Part model, mm, in its own coordinate system. A direction names the side the tool comes from. Coordinates: 2 decimals unless noted, no trailing zeros. Loops run counter-clockwise (first coordinate to the right, second up) from the corner with the lowest first, then second, coordinate; pieces in that order, holes last.
```python
from build123d import *

# Parameters (mm, degrees)
EXTRUDE_1_DEPTH       = 200
SKETCH_3_W            = 148
SKETCH_3_H            = 194
CUT_EXTRUDE_1_DEPTH   = 44
SKETCH_4_W            = 8
SKETCH_4_H            = 194
EXTRUDE_1_2_DEPTH     = 44
CUT_EXTRUDE_2_DEPTH   = 222.580685079
CUT_EXTRUDE_5_DEPTH   = 219.876677606
MOVE_FACE_1_BY        = 2
MOVE_FACE_1_2_BY      = 2
CUT_EXTRUDE_6_DEPTH   = 222.580685079
CUT_EXTRUDE_7_DEPTH   = 16.595837
MOVE_FACE_2_BY        = 45
MOVE_FACE_3_BY        = 20
SKETCH_13_W           = 71
SKETCH_13_H           = 47
CUT_EXTRUDE_8_DEPTH   = 25
SKETCH_14_W           = 69
SKETCH_14_H           = 26
CUT_EXTRUDE_9_DEPTH   = 45
CUT_EXTRUDE_10_DEPTH  = 45
CHAMFER_1_SIZE        = 25
CUT_EXTRUDE_11_REACH  = 222.964
SKETCH_16_W           = 71
SKETCH_16_H           = 85
SKETCH_17_W           = 71
SKETCH_17_H           = 3
EXTRUDE_2_DEPTH       = 10
SKETCH_18_W           = 18.7
SKETCH_18_H           = 5
CUT_EXTRUDE_12_DEPTH  = 2.2
SKETCH_19_W           = 69
SKETCH_19_H           = 90
EXTRUDE_3_DEPTH       = 15
SKETCH_20_W           = 56
SKETCH_20_H           = 87
CUT_EXTRUDE_13_DEPTH  = 10
CUT_EXTRUDE_14_REACH  = 220.472
SKETCH_21_W           = 36
SKETCH_21_H           = 34
SKETCH_22_W           = 2
SKETCH_22_H           = 17
SKETCH_22_H_2         = 35
CUT_EXTRUDE_1_2_DEPTH = 7
MOVE_FACE_4_BY        = 3
CHAMFER_2_SIZE        = 1


with BuildPart() as part:
    # 草图1 → Extrude 1 (new body)
    with BuildSketch(Plane.XY):
        Polygon((77, 0), (-77, 0), (-77, 31), (-83, 37), (-83, 41), (-77, 47), (77, 47), (83, 41), (83, 37), (77, 31), align=None)
    extrude(amount=-EXTRUDE_1_DEPTH)

    # 草图3 → Cut-Extrude 1 (cut)
    with BuildSketch(Plane(origin=(0, 47, 0), x_dir=(1, 0, 0), z_dir=(0, 1, 0))):
        with Locations((0, 100)):
            Rectangle(SKETCH_3_W, SKETCH_3_H)
    extrude(amount=-CUT_EXTRUDE_1_DEPTH, mode=Mode.SUBTRACT)

    # 草图4 → Extrude 1 2 (add)
    with BuildSketch(Plane(origin=(0, 3, 0), x_dir=(1, 0, 0), z_dir=(0, 1, 0))):
        with Locations((1, 100)):
            Rectangle(SKETCH_4_W, SKETCH_4_H)
    extrude(amount=EXTRUDE_1_2_DEPTH)

    # 草图5 → 切除-拉伸2 (cut, through all)
    with BuildSketch(Plane(origin=(0, 0, -200), x_dir=(-1, 0, 0), z_dir=(0, 0, -1))):
        Polygon((-74, 47), (-74, 44.767409819), (-79, 39.767409819), (-79, 38.656854249), (-74, 33.656854249), (-74, 26), (-5, 26), (-5, 33.656854249), (0, 38.656854249), (0, 39.767409819), (-5, 44.767409819), (-5, 47), align=None)
    extrude(amount=-CUT_EXTRUDE_2_DEPTH, mode=Mode.SUBTRACT)

    # 草图9 → 切除-拉伸5 (cut, through all)
    with BuildSketch(Plane(origin=(0, 0, -3), x_dir=(-1, 0, 0), z_dir=(0, 0, -1))):
        Polygon((-4.404163056, 47), (3, 39.595836944), (74, 39.595836944), (74, 47), (3, 47), align=None)
    extrude(amount=CUT_EXTRUDE_5_DEPTH, mode=Mode.SUBTRACT)

    # Move Face 1: a face moved outward by 2.0
    extrude(part.faces().sort_by_distance((39.5, 14.5, -197))[0], amount=MOVE_FACE_1_BY, dir=(0, 0, 1))

    # Move Face 1 2: a face moved outward by 2.0
    extrude(part.faces().sort_by_distance((-38.5, 21.297918472, -197))[0], amount=MOVE_FACE_1_2_BY, dir=(0, 0, 1))

    # 草图11 → 切除-拉伸6 (cut, through all)
    with BuildSketch(Plane.XZ):
        Polygon((51.883419246, -200), (53.904145188, -196.5), (23.095854812, -196.5), (25.116580754, -200), align=None)
        Polygon((-53.904145188, -196.5), (-23.095854812, -196.5), (-25.116580754, -200), (-51.883419246, -200), align=None)
    extrude(amount=-CUT_EXTRUDE_6_DEPTH, mode=Mode.SUBTRACT)

    # 草图12 → 切除-拉伸7 (cut)
    with BuildSketch(Plane(origin=(0, 39.595836944, 0), x_dir=(1, 0, 0), z_dir=(0, 1, 0))):
        Polygon((-53.904145188, 196.5), (-51.883419246, 200), (-74, 200), (-74, 195), (-3, 195), (-3, 200), (-25.116580754, 200), (-23.095854812, 196.5), align=None)
        Polygon((53.904145188, 196.5), (23.095854812, 196.5), (25.116580754, 200), (5, 200), (5, 195), (74, 195), (74, 200), (51.883419246, 200), align=None)
    extrude(amount=-CUT_EXTRUDE_7_DEPTH, mode=Mode.SUBTRACT)

    # Move Face 2: a face moved outward by 45.0
    extrude(part.faces().sort_by_distance((-10.200110487, 20.43272532, 0))[0], amount=MOVE_FACE_2_BY, dir=(0, 0, 1))

    # Move Face 3: a face moved inward by 20.0
    extrude(part.faces().sort_by_distance((-38.169755743, 25.169887896, -3))[0], amount=MOVE_FACE_3_BY, dir=(0, 0, 1), mode=Mode.SUBTRACT)

    # 草图13 → 切除-拉伸8 (cut)
    with BuildSketch(Plane.XY.offset(45)):
        with Locations((-38.5, 23.5)):
            Rectangle(SKETCH_13_W, SKETCH_13_H)
    extrude(amount=-CUT_EXTRUDE_8_DEPTH, mode=Mode.SUBTRACT)

    # 草图14 → 切除-拉伸9 (cut)
    with BuildSketch(Plane.XY.offset(45)):
        with Locations((39.5, 13)):
            Rectangle(SKETCH_14_W, SKETCH_14_H)
    extrude(amount=-CUT_EXTRUDE_9_DEPTH, mode=Mode.SUBTRACT)

    # 草图15 → 切除-拉伸10 (cut)
    with BuildSketch(Plane.XY.offset(45)):
        Polygon((5, 0), (0, 0), (0, 25.656854249), (5, 30.656854249), align=None)
    extrude(amount=-CUT_EXTRUDE_10_DEPTH, mode=Mode.SUBTRACT)

    # 倒角1
    chamfer_1_edges = [part.edges().sort_by_distance(p)[0] for p in [
        (75.5, 0, 45),
        (-1.5, 0, 45),
        (-75.5, 0, 45),
    ]]
    chamfer(chamfer_1_edges, length=CHAMFER_1_SIZE)

    # 草图16 → 切除-拉伸11 (cut, up to next)
    with BuildSketch(Plane(origin=(0, 3, 0), x_dir=(1, 0, 0), z_dir=(0, 1, 0)), mode=Mode.PRIVATE) as cut_extrude_11_sk1:
        with Locations((-38.5, 152.5)):
            Rectangle(SKETCH_16_W, SKETCH_16_H)
    cut_extrude_11_tool1 = extrude(cut_extrude_11_sk1.sketch, amount=-CUT_EXTRUDE_11_REACH, mode=Mode.PRIVATE) & part.part
    add(cut_extrude_11_tool1.solids().sort_by_distance((-38.5, 3, -152.5))[0], mode=Mode.SUBTRACT)

    # 草图17 → 凸台-拉伸2 (add)
    with BuildSketch(Plane(origin=(0, 3, 0), x_dir=(1, 0, 0), z_dir=(0, 1, 0))):
        with Locations((-38.5, 108.5)):
            Rectangle(SKETCH_17_W, SKETCH_17_H)
    extrude(amount=EXTRUDE_2_DEPTH)

    # 草图18 → 切除-拉伸12 (cut)
    with BuildSketch(Plane(origin=(0, 23, 0), x_dir=(1, 0, 0), z_dir=(0, 1, 0))):
        with Locations((-12.35, 197.5)):
            Rectangle(SKETCH_18_W, SKETCH_18_H)
        with Locations((-64.65, 197.5)):
            Rectangle(SKETCH_18_W, SKETCH_18_H)
    extrude(amount=-CUT_EXTRUDE_12_DEPTH, mode=Mode.SUBTRACT)

    # 草图19 → 凸台-拉伸3 (add)
    with BuildSketch(Plane(origin=(0, 3, 0), x_dir=(1, 0, 0), z_dir=(0, 1, 0))):
        with Locations((39.5, 150)):
            Rectangle(SKETCH_19_W, SKETCH_19_H)
    extrude(amount=EXTRUDE_3_DEPTH)

    # 草图20 → 切除-拉伸13 (cut)
    with BuildSketch(Plane(origin=(0, 18, 0), x_dir=(1, 0, 0), z_dir=(0, 1, 0))):
        with Locations((33, 151.5)):
            Rectangle(SKETCH_20_W, SKETCH_20_H)
    extrude(amount=-CUT_EXTRUDE_13_DEPTH, mode=Mode.SUBTRACT)

    # 切除-拉伸14: up to this face of the body (flat: up to its plane)
    cut_extrude_14_end = Plane(part.part.faces().sort_by_distance((39.5, 3, -54))[0])
    # 草图21 → 切除-拉伸14 (cut, up to the picked face)
    with BuildSketch(Plane(origin=(0, 18, 0), x_dir=(1, 0, 0), z_dir=(0, 1, 0)), mode=Mode.PRIVATE) as cut_extrude_14_sk1:
        with Locations((33, 108)):
            Rectangle(SKETCH_21_W, SKETCH_21_H)
    cut_extrude_14_tool1 = split(extrude(cut_extrude_14_sk1.sketch, amount=-CUT_EXTRUDE_14_REACH, mode=Mode.PRIVATE), bisect_by=cut_extrude_14_end, keep=Keep.BOTH, mode=Mode.PRIVATE)
    add(cut_extrude_14_tool1.solids().sort_by(Axis((33, 18, -108), (0, -1, 0)))[0], mode=Mode.SUBTRACT)

    # 草图22 → Cut-Extrude 1 2 (cut)
    with BuildSketch(Plane(origin=(0, 18, 0), x_dir=(1, 0, 0), z_dir=(0, 1, 0))):
        with Locations((66, 181.5)):
            Rectangle(SKETCH_22_W, SKETCH_22_H)
        with Locations((66, 158.5)):
            Rectangle(SKETCH_22_W, SKETCH_22_H)
        with Locations((66, 126.5)):
            Rectangle(SKETCH_22_W, SKETCH_22_H_2)
    extrude(amount=-CUT_EXTRUDE_1_2_DEPTH, mode=Mode.SUBTRACT)

    # Move Face 4: a face moved outward by 3.0
    extrude(part.faces().sort_by_distance((66, 11, -126.5))[0], amount=MOVE_FACE_4_BY, dir=(0, 1, 0))

    # 倒角2
    chamfer_2_edges = [part.edges().sort_by_distance(p)[0] for p in [
        (-80, 34, 45),
        (-83, 39, 45),
        (-80, 44, 45),
        (80, 44, 45),
        (83, 39, 45),
        (80, 34, 45),
        (80, 34, -200),
        (83, 39, -200),
        (80, 44, -200),
        (-80, 44, -200),
        (-83, 39, -200),
        (-80, 34, -200),
        (2.5, 42.267409819, 45),
        (0, 39.212132034, 45),
        (2.5, 36.156854249, 45),
        (76.5, 36.156854249, 45),
        (79, 39.212132034, 45),
        (76.5, 42.267409819, 45),
        (76.5, 42.267409819, -200),
        (76.5, 36.156854249, -200),
        (2.5, 36.156854249, -200),
        (0, 39.212132034, -200),
        (2.5, 42.267409819, -200),
    ]]
    chamfer(chamfer_2_edges, length=CHAMFER_2_SIZE)


solid = part.part
```
Q1. Tool access for faces 5 (the flat face through (77, 16, -79)), 6 (the flat face through (76.545, 35.485, -199.507)), 7 (the flat face through (-65, 20.8, -198)), 8 (the flat face through (2.4, 35.56, 44.49)), 9 (the flat face through (31, 16, -195)): list every direction of +Z, -Z, +X, -X, +Y, -Y with a clear straight run to the whole face (end or side of a thin tool).
Q2. Saw through at D-D (x = -33). List the corners of the cut face in (y, z), plus the area to 4 significant figures.
Q3. Probe line 1 (X direction, y = 25.5, z = -134); line 2 (X direction, y = 10, z = -187); line 3 (Z direction, x = 33.5, y = 13.5). List the from-to ranges inside material, lowest first.
Q4. Saw through at C-C (z = -87). List the corners of the cut face in (x, y), plus the area to 3 significant figures.
Q5. Saw through at B-B (x = 9). List the corners of the cut face in (y, z).
Q6. Saw through at A-A (x = -11.5). List the corners of the cut face in (y, z), plus the area to 3 significant figures.
Q7. Drop flat-ended pins along their axis: P1, Ø0.6, axis at x = 66, z = -162, coming from the +Y side; P2, Ø1.1, axis at y = 46, z = -17.5, coming from the +X side; P3, Ø7, axis at x = 34.5, y = 13, coming from the -Z side; P4, Ø12, axis at x = -9.5, z = -123, coming from the -Y side. Give the stop position or say it passes through.
Q8. Mould opens along Z. For faces 1 (the flat face through (0, 13, -200)), 2 (the flat face through (-79.345, 43.958, 44.493)), 3 (the flat face through (0.754, 43.35, -93.019)), 4 (the flat face through (-39, 7, -110)) say: released by +Z, released by -Z, zero draft, split by the parting line, or undercut.
Checked values:
1. face 5: +Z, -Z, +X, -Y
1. face 6: -Z
1. face 7: -Z, +Y
1. face 8: +Z
1. face 9: +Y
2. outline: (0, -196.5) - (23, -196.5) - (23, -195) - (0, -195) - close; (0, -110) - (13, -110) - (13, -107) - (3, -107) - (3, 17) - (47, 17) - (47, 20) - (0, 20) - close
2. area: 586.5 mm2
3. line 1: x = -77 to -74, -3 to 5, 74 to 77
3. line 2: x = -77 to -74, -3 to 5, 61 to 77
3. line 3: z = -196.5 to -195, -3 to 0
4. outline: (-83, 37) - (-77, 31) - (-77, 0) - (77, 0) - (77, 31) - (83, 37) - (83, 41) - (77, 47) - (74, 47) - (74, 44.77) - (79, 39.77) - (79, 38.66) - (74, 33.66) - (74, 3) - (5, 3) - (5, 33.66) - (0, 38.66) - (0, 39.77) - (5, 44.77) - (5, 47) - (4.4, 47) - (-3, 39.6) - (-3, 3) - (-74, 3) - (-74, 47) - (-77, 47) - (-83, 41) - close
4. area: 1,110 mm2
5. outline: (0, -200) - (23, -200) - (23, -195) - (8, -195) - (8, -108) - (18, -108) - (18, -105) - (3, -105) - (3, -3) - (26, -3) - (26, 0) - (0, 0) - close
6. outline: (0, -200) - (20.8, -200) - (20.8, -195) - (0, -195) - close; (0, -110) - (13, -110) - (13, -107) - (3, -107) - (3, 17) - (47, 17) - (47, 20) - (0, 20) - close
6. area: 656 mm2
7. P1: stops at y = 11
7. P2: stops at x = 78.55
7. P3: stops at z = -196.5
7. P4: passes through
8. face 1: released by -Z
8. face 2: released by +Z
8. face 3: zero draft
8. face 4: undercut
